Geometry: final body of the model. Coordinates: model frame, mm. A direction names the side the tool comes from. Coordinates: 2 decimals unless noted, no trailing zeros. Loops run counter-clockwise (first coordinate to the right, second up) from the corner with the lowest first, then second, coordinate; pieces in that order, holes last. Notation, with made-up numbers: (-32, -2.5) - (-2, -2.5) arc R24 ccw to (-2, 33.5) - close; hole circle Ø11 at (-29, 50.5). An arc over 180 degrees is marked (long way). Return JSON: item names as keys, results as strings.
from build123d import *

# Parameters (mm, degrees)
RESSALTO_EXTRUS_O1_DEPTH = 18
ESBO_O2_R                = 1.75
ESBO_O2_R_2              = 2
CORTE_EXTRUS_O1_DEPTH    = 43.118879377


with BuildPart() as part:
    # Esboço1 → Ressalto-extrusão1 (new body)
    with BuildSketch(Plane.XY):
        Polygon((-35, 0), (-25, 0), (-25, 12.5), (-10, 12.5), (-10, 0), (0, 0), (0, -2.5), (-12.5, -2.5), (-12.5, 10), (-22.5, 10), (-22.5, -2.5), (-35, -2.5), align=None)
    extrude(amount=RESSALTO_EXTRUS_O1_DEPTH)

    # Esboço2 → Corte-extrusão1 (cut, through all)
    with BuildSketch(Plane(origin=(0, 12.5, 0), x_dir=(1, 0, 0), z_dir=(0, 1, 0))):
        with Locations(Location((-17.5, -4.3, 0), (0, 0, 270))):
            Circle(ESBO_O2_R)
        with Locations(Location((-30, -9, 0), (0, 0, 270))):
            Circle(ESBO_O2_R_2)
        with Locations(Location((-5, -9, 0), (0, 0, 90))):
            Circle(ESBO_O2_R_2)
        with BuildLine():
            Line((-19.25, -14.7), (-19.25, -12.7))
            ThreePointArc((-19.25, -12.7), (-17.5, -10.95), (-15.75, -12.7))
            Line((-15.75, -12.7), (-15.75, -14.7))
            ThreePointArc((-15.75, -14.7), (-17.5, -16.45), (-19.25, -14.7))
        make_face()
    extrude(amount=-CORTE_EXTRUS_O1_DEPTH, mode=Mode.SUBTRACT)


solid = part.part
Item 1: Section query B-B, the plane z = 13.25. Return loops of the section in (x, y).
Worked out:
{"outline": "(-35, -2.5) - (-22.5, -2.5) - (-22.5, 10) - (-19.25, 10) - (-19.25, 12.5) - (-25, 12.5) - (-25, 0) - (-35, 0) - close; (-15.75, 10) - (-12.5, 10) - (-12.5, -2.5) - (0, -2.5) - (0, 0) - (-10, 0) - (-10, 12.5) - (-15.75, 12.5) - close"}
Item 2: Section query A-A, the plane y = -1.25. Return loops of the section in (x, z), and give its area (3 significant figures).
Worked out:
{"outline": "(-35, 0) - (-22.5, 0) - (-22.5, 18) - (-35, 18) - close; (-12.5, 0) - (0, 0) - (0, 18) - (-12.5, 18) - close; hole circle Ø4 at (-30, 9); hole circle Ø4 at (-5, 9)", "area": "425 mm^2"}
Item 3: Mould query, pull axis X, two halves, no side actions, for faces 1 (the face through (-12, 4, 18)), 2 (the face through (-15.765, 11.268, 4.072)), 3 (the face through (-10, 6, 9)). Classes: +X half, -X half, draft (parallel to the pull), parting line (faces both ways), or undercut.
Worked out:
{"face 1": "draft", "face 2": "undercut", "face 3": "+X half"}
Item 4: Reachability of faces 4 (the face through (-27.8, 0, 8.9)), 5 (the face through (-17.46, 11.27, 16.45)), 6 (the face through (-2.8, 0, 8.9)), 7 (the face through (-12.5, 4, 9)) from +Z, -Z, +X, -X, +Y, -Y: full face, straight path, thin tool, end or side. Return the list, or none.
Worked out:
{"face 4": "+Z, -Z, -X, +Y", "face 5": "+Y, -Y", "face 6": "+Z, -Z, +X, +Y", "face 7": "+Z, -Z, -Y"}
Item 5: Section query C-C, the plane x = -30. Return loops of the section in (y, z).
Worked out:
{"outline": "(-2.5, 0) - (0, 0) - (0, 7) - (-2.5, 7) - close; (-2.5, 11) - (0, 11) - (0, 18) - (-2.5, 18) - close"}
Item 6: First-contact query: pin 1 Ø4 at (y, z) = (8.5, 6) entering from +X; pin 2 Ø4.5 at (x, z) = (-17.5, 4.3) entering from -Y; pin 3 Ø8 at (x, z) = (-3, 13.5) entering from +Y. Flat tips, straight axial feed; report the tip coordinate or a pass-through.
Worked out:
{"pin 1": "x = -10", "pin 2": "y = 10", "pin 3": "y = 0"}
Item 7: Section query D-D, the plane y = 1.25. Return loops of the section in (x, z).
Worked out:
{"outline": "(-25, 0) - (-22.5, 0) - (-22.5, 18) - (-25, 18) - close; (-12.5, 0) - (-10, 0) - (-10, 18) - (-12.5, 18) - close"}
Item 8: Ray query, probe 1 along X at (y, z) = (-1.55, 9); probe 2 along X at (y, z) = (2.75, 4); probe 3 along Z at (x, y) = (-5, -1). Return the intervals inside material, ascending. Write a range as from..to.
Worked out:
{"probe 1": "-35..-32, -28..-22.5, -12.5..-7, -3..0", "probe 2": "-25..-22.5, -12.5..-10", "probe 3": "0..7, 11..18"}
